Geometry: final body of the model. Coordinates: model frame, mm. A direction names the side the tool comes from. Give positions to 0.01 mm unless a question says otherwise; leave off trailing zeros. Loops run counter-clockwise (first coordinate to the right, second up) from the corner with the lowest first, then second, coordinate; pieces in that order, holes last.
from build123d import *

# Parameters (mm, degrees)
SKETCH1_W           = 419.1
SKETCH1_H           = 142.18412
BOSS_EXTRUDE1_DEPTH = 88.9
SKETCH2_R           = 119.38
CUT_EXTRUDE1_DEPTH  = 83.4009
SKETCH7_W           = 187.160719179
SKETCH7_H           = 30.93974
SKETCH7_H_2         = 43.28668
CUT_EXTRUDE2_DEPTH  = 452.402640644
SKETCH4_R           = 40.386
CUT_EXTRUDE4_DEPTH  = 7.62
CUT_EXTRUDE17_START = -12.7
CUT_EXTRUDE17_DEPTH = 12.7
CUT_EXTRUDE18_DEPTH = 12.7
SKETCH18_R          = 25.527
CUT_EXTRUDE11_DEPTH = 23.09114
SKETCH8_W           = 419.1
SKETCH8_H           = 88.9
CUT_EXTRUDE6_DEPTH  = 7.85114
SKETCH9_W           = 419.1
SKETCH9_H           = 88.9
CUT_EXTRUDE7_DEPTH  = 7.14248
SKETCH10_W          = 219.202
SKETCH10_H          = 88.9
CUT_EXTRUDE8_DEPTH  = 30.48
SKETCH12_W          = 121.533574186
SKETCH12_H          = 96.7105
BOSS_EXTRUDE2_DEPTH = 50.8
SKETCH14_W          = 55.647095764
SKETCH14_H          = 96.7105
BOSS_EXTRUDE3_DEPTH = 12.7
CUT_EXTRUDE10_REACH = 448.907
SKETCH17_R          = 12.827
SKETCH22_W          = 199.898
SKETCH22_H          = 88.9
BOSS_EXTRUDE5_DEPTH = 2.54
SKETCH29_R          = 12.827
CUT_EXTRUDE14_DEPTH = 447.906526346
BOSS_EXTRUDE6_DEPTH = 86.10092
SKETCH45_W          = 107.95
SKETCH45_H          = 50.53076
SKETCH45_H_2        = 15.24
CUT_EXTRUDE22_DEPTH = 452.677672269
SKETCH46_W          = 91.948
SKETCH46_H          = 129.7305
BOSS_EXTRUDE7_DEPTH = 12.7
CUT_EXTRUDE23_DEPTH = 452.677672176


with BuildPart() as part:
    # Sketch1 → Boss-Extrude1 (new body)
    with BuildSketch(Plane(origin=(0, 0, 0), x_dir=(1, 0, 0), z_dir=(0, 1, 0))):
        with Locations((209.55, 71.09206)):
            Rectangle(SKETCH1_W, SKETCH1_H)
    extrude(amount=BOSS_EXTRUDE1_DEPTH)

    # Sketch2 → Cut-Extrude1 (cut)
    with BuildSketch(Plane(origin=(0, 0, -131.63296), x_dir=(-1, 0, 0), z_dir=(0, 0, -1))):
        with Locations((-116.7166499, 150.061217688)):
            Circle(SKETCH2_R)
    extrude(amount=-CUT_EXTRUDE1_DEPTH, mode=Mode.SUBTRACT)

    # Sketch7 → Cut-Extrude2 (cut, through all)
    with BuildSketch(Plane(origin=(0, 88.9, 0), x_dir=(1, 0, 0), z_dir=(0, 1, 0))):
        with Locations((325.519640411, 103.62311)):
            Rectangle(SKETCH7_W, SKETCH7_H)
        with Locations((325.519640411, 33.4899)):
            Rectangle(SKETCH7_W, SKETCH7_H_2)
    extrude(amount=-CUT_EXTRUDE2_DEPTH, mode=Mode.SUBTRACT)

    # Sketch4 → Cut-Extrude4 (cut)
    with BuildSketch(Plane(origin=(0, 0, -67.83324), x_dir=(-1, 0, 0), z_dir=(0, 0, -1))):
        with Locations((-278.649352085, 104.852009966)):
            Circle(SKETCH4_R)
    extrude(amount=CUT_EXTRUDE4_DEPTH, mode=Mode.SUBTRACT)

    # Sketch39 → Cut-Extrude17 (cut)
    with BuildSketch(Plane.XY.offset(-55.13324).offset(CUT_EXTRUDE17_START)):
        with BuildLine():
            Line((231.939280821, 58.527426444), (231.939280821, 88.9))
            Line((231.939280821, 88.9), (342.472006166, 88.9))
            ThreePointArc((342.472006166, 88.9), (296.080170447, 41.417284719), (231.939280821, 58.527426444))
        make_face()
    extrude(amount=CUT_EXTRUDE17_DEPTH, mode=Mode.SUBTRACT)

    # Sketch40 → Cut-Extrude18 (cut)
    with BuildSketch(Plane(origin=(0, 0, -88.15324), x_dir=(-1, 0, 0), z_dir=(0, 0, -1))):
        with BuildLine():
            Line((-231.939280821, 88.9), (-231.939280821, 58.527426444))
            ThreePointArc((-231.939280821, 58.527426444), (-296.080170447, 41.417284719), (-342.472006166, 88.9))
            Line((-342.472006166, 88.9), (-231.939280821, 88.9))
        make_face()
    extrude(amount=-CUT_EXTRUDE18_DEPTH, mode=Mode.SUBTRACT)

    # Sketch18 → Cut-Extrude11 (cut)
    with BuildSketch(Plane(origin=(0, 0, -142.18412), x_dir=(-1, 0, 0), z_dir=(0, 0, -1))):
        with Locations((-278.649352085, 104.852009966)):
            Circle(SKETCH18_R)
    extrude(amount=-CUT_EXTRUDE11_DEPTH, mode=Mode.SUBTRACT)

    # Sketch8 → Cut-Extrude6 (cut)
    with BuildSketch(Plane(origin=(0, 0, -142.18412), x_dir=(-1, 0, 0), z_dir=(0, 0, -1))):
        with Locations((-209.55, 44.45)):
            Rectangle(SKETCH8_W, SKETCH8_H)
    extrude(amount=-CUT_EXTRUDE6_DEPTH, mode=Mode.SUBTRACT)

    # Sketch9 → Cut-Extrude7 (cut)
    with BuildSketch(Plane.XY):
        with Locations((209.55, 44.45)):
            Rectangle(SKETCH9_W, SKETCH9_H)
    extrude(amount=-CUT_EXTRUDE7_DEPTH, mode=Mode.SUBTRACT)

    # Sketch10 → Cut-Extrude8 (cut)
    with BuildSketch(Plane.XY.offset(-7.14248)):
        with Locations((109.601, 44.45)):
            Rectangle(SKETCH10_W, SKETCH10_H)
    extrude(amount=-CUT_EXTRUDE8_DEPTH, mode=Mode.SUBTRACT)

    # Sketch12 → Boss-Extrude2 (add)
    with BuildSketch(Plane.XZ):
        with Locations((-60.766787093, -85.97773)):
            Rectangle(SKETCH12_W, SKETCH12_H)
    extrude(amount=-BOSS_EXTRUDE2_DEPTH)

    # Sketch14 → Boss-Extrude3 (add)
    with BuildSketch(Plane.XZ):
        with Locations((-93.710026304, -85.97773)):
            Rectangle(SKETCH14_W, SKETCH14_H)
    extrude(amount=BOSS_EXTRUDE3_DEPTH)

    # Cut-Extrude10: up to this face of the body (flat: up to its plane)
    cut_extrude10_end = Plane(part.part.faces().sort_by_distance((319.151, 44.45, -7.14248))[0])
    # Sketch17 → Cut-Extrude10 (cut, up to the picked face)
    with BuildSketch(Plane(origin=(0, 0, -134.33298), x_dir=(-1, 0, 0), z_dir=(0, 0, -1)), mode=Mode.PRIVATE) as cut_extrude10_sk1:
        with Locations((-384.735935495, 0.531880938)):
            Circle(SKETCH17_R)
    cut_extrude10_tool1 = split(extrude(cut_extrude10_sk1.sketch, amount=-CUT_EXTRUDE10_REACH, mode=Mode.PRIVATE), bisect_by=cut_extrude10_end, keep=Keep.BOTH, mode=Mode.PRIVATE)
    # Sketch17 → Cut-Extrude10 (cut, up to the picked face)
    with BuildSketch(Plane(origin=(0, 0, -134.33298), x_dir=(-1, 0, 0), z_dir=(0, 0, -1)), mode=Mode.PRIVATE) as cut_extrude10_sk2:
        with Locations((94.798916194, -17.274045482)):
            Circle(SKETCH17_R)
    cut_extrude10_tool2 = split(extrude(cut_extrude10_sk2.sketch, amount=-CUT_EXTRUDE10_REACH, mode=Mode.PRIVATE), bisect_by=cut_extrude10_end, keep=Keep.BOTH, mode=Mode.PRIVATE)
    # Sketch17 → Cut-Extrude10 (cut, up to the picked face)
    with BuildSketch(Plane(origin=(0, 0, -134.33298), x_dir=(-1, 0, 0), z_dir=(0, 0, -1)), mode=Mode.PRIVATE) as cut_extrude10_sk3:
        with BuildLine():
            Line((-169.736021607, 19.31637742), (-169.736021607, 0))
            Line((-169.736021607, 0), (-144.082021607, 0))
            Line((-144.082021607, 0), (-144.082021607, 19.31637742))
            ThreePointArc((-144.082021607, 19.31637742), (-156.909021607, 32.14337742), (-169.736021607, 19.31637742))
        make_face()
    cut_extrude10_tool3 = split(extrude(cut_extrude10_sk3.sketch, amount=-CUT_EXTRUDE10_REACH, mode=Mode.PRIVATE), bisect_by=cut_extrude10_end, keep=Keep.BOTH, mode=Mode.PRIVATE)
    add(cut_extrude10_tool1.solids().sort_by(Axis((384.735935, 0.531881, -134.33298), (0, 0, 1)))[0], mode=Mode.SUBTRACT)
    add(cut_extrude10_tool2.solids().sort_by(Axis((-94.798916, -17.274045, -134.33298), (0, 0, 1)))[0], mode=Mode.SUBTRACT)
    add(cut_extrude10_tool3.solids().sort_by(Axis((156.909022, 14.834778, -134.33298), (0, 0, 1)))[0], mode=Mode.SUBTRACT)

    # Sketch22 → Boss-Extrude5 (add)
    with BuildSketch(Plane.XY.offset(-7.14248)):
        with Locations((319.151, 44.45)):
            Rectangle(SKETCH22_W, SKETCH22_H)
    extrude(amount=BOSS_EXTRUDE5_DEPTH)

    # Sketch29 → Cut-Extrude14 (cut, through all)
    with BuildSketch(Plane(origin=(0, 0, -7.14248), x_dir=(-1, 0, 0), z_dir=(0, 0, -1))):
        with Locations((-384.735935495, 0.531880938)):
            Circle(SKETCH29_R)
    extrude(amount=-CUT_EXTRUDE14_DEPTH, mode=Mode.SUBTRACT)

    # Sketch30 → Boss-Extrude6 (add)
    with BuildSketch(Plane(origin=(0, 0, -134.33298), x_dir=(-1, 0, 0), z_dir=(0, 0, -1))):
        with BuildLine():
            Line((-14.194018979, 88.9), (-20.758717893, 88.9))
            ThreePointArc((-20.758717893, 88.9), (-116.7166499, 36.269217688), (-212.674581906, 88.9))
            Line((-212.674581906, 88.9), (-219.239280821, 88.9))
            ThreePointArc((-219.239280821, 88.9), (-116.7166499, 30.681217688), (-14.194018979, 88.9))
        make_face()
    extrude(amount=-BOSS_EXTRUDE6_DEPTH)

    # Sketch44 → Cut-Revolve1 (revolve, cut)
    with BuildSketch(Plane(origin=(0, 104.852009966, 0), x_dir=(1, 0, 0), z_dir=(0, 1, 0))):
        with BuildLine():
            Line((278.649352085, 11.84656), (306.589352085, 11.84656))
            ThreePointArc((306.589352085, 11.84656), (307.31205993, 7.964449393), (309.383352085, 4.60248))
            Line((309.383352085, 4.60248), (278.649352085, 4.60248))
            Line((278.649352085, 4.60248), (278.649352085, 11.84656))
        make_face()
    revolve(axis=Axis((278.649352085, 104.852009966, -328.456473898), (0, 0, 1)), mode=Mode.SUBTRACT)

    # Sketch45 → Cut-Extrude22 (cut, through all)
    with BuildSketch(Plane(origin=(0, 88.9, 0), x_dir=(1, 0, 0), z_dir=(0, 1, 0))):
        with Locations((365.125, 29.86786)):
            Rectangle(SKETCH45_W, SKETCH45_H)
        with Locations((365.125, 126.71298)):
            Rectangle(SKETCH45_W, SKETCH45_H_2)
    extrude(amount=-CUT_EXTRUDE22_DEPTH, mode=Mode.SUBTRACT)

    # Sketch46 → Boss-Extrude7 (add)
    with BuildSketch(Plane.XZ):
        with Locations((265.176, -69.46773)):
            Rectangle(SKETCH46_W, SKETCH46_H)
    extrude(amount=-BOSS_EXTRUDE7_DEPTH)

    # Sketch47 → Cut-Extrude23 (cut, through all)
    with BuildSketch(Plane(origin=(0, 88.9, 0), x_dir=(1, 0, 0), z_dir=(0, 1, 0))):
        with BuildLine():
            Line((222.900157375, 134.33298), (90.917885838, 134.33298))
            ThreePointArc((90.917885838, 134.33298), (156.909021607, 96.23298), (222.900157375, 134.33298))
        make_face()
    extrude(amount=-CUT_EXTRUDE23_DEPTH, mode=Mode.SUBTRACT)


solid = part.part
Item 1: Draft query along X for faces 5 (the face through (311.15, 35, -121)), 6 (the face through (271, 12.7, -103)), 7 (the face through (-95.02, -4.45, -86.65)). Return one class per face: +X half, -X half, draft (parallel to the pull), parting line (faces both ways), or undercut.
Values follow:
face 5: +X half
face 6: draft
face 7: undercut
Item 2: Section query C-C on z = -27. Return loops of the section in (x, y).
Values follow:
outline: (219.2, 0) - (311.15, 0) - (311.15, 12.7) - (231.94, 12.7) - (231.94, 88.9) - (219.2, 88.9) - close
Item 3: Section query D-D on x = -43. Return loops of the section in (y, z).
Values follow:
outline: (0, -134.33) - (50.8, -134.33) - (50.8, -37.62) - (0, -37.62) - close
Item 4: Section query A-A on z = -102.5. Return loops of the section in (x, y), plus the area to 3 significant figures.
Values follow:
outline: (-121.53, -12.7) - (-106.78, -12.7) arc R12.83 cw to (-82.82, -12.7) - (-65.89, -12.7) - (-65.89, 0) - (126.65, 0) - (126.65, 36.7) arc R113.79 cw to (20.76, 88.9) - (0, 88.9) - (0, 50.8) - (-121.53, 50.8) - close; (187.17, 0) - (311.15, 0) - (311.15, 12.7) - (231.94, 12.7) - (231.94, 88.9) - (212.67, 88.9) arc R113.79 cw to (187.17, 60.7) - close
area: 18,500 mm2
Item 5: Ray query, probe 1 along Z at (x, y) = (232.5, 56); probe 2 along Z at (x, y) = (245, 67); probe 3 along X at (y, z) = (14, -48). Return the intervals inside material, ascending.
Values follow:
probe 1: z = -134.33 to -119.09, -88.15 to -55.13, -11.85 to -4.6
probe 2: z = -134.33 to -119.09, -75.45 to -67.83, -11.85 to -4.6
probe 3: x = -121.53 to 144.08, 169.74 to 231.94
Item 6: Pin query (flat end, axial travel): pin 1 (19 mm diameter, centred on y = 74.5, z = -64.5, fed in from -X); pin 2 (4 mm diameter, centred on y = 28.5, z = -26.5, fed in from +X); pin 3 (4 mm diameter, centred on x = 184.5, z = -46, fed in from -Y). Return the tip coordinate at first contact, or that it passes through.
Values follow:
pin 1: stops at x = 0
pin 2: stops at x = 231.94
pin 3: stops at y = 0
Item 7: Section query B-B on y = 6. Return loops of the section in (x, z).
Values follow:
outline: (-121.53, -134.33) - (90.92, -134.33) arc R76.2 cw to (144.08, -97.32) - (144.08, -37.62) - (-121.53, -37.62) - close; (169.74, -97.32) arc R76.2 cw to (222.9, -134.33) - (311.15, -134.33) - (311.15, -88.15) - (373.13, -88.15) - (373.13, -55.13) - (311.15, -55.13) - (311.15, -4.6) - (219.2, -4.6) - (219.2, -37.62) - (169.74, -37.62) - close; (396.34, -88.15) - (419.1, -88.15) - (419.1, -55.13) - (396.34, -55.13) - close
Item 8: Set-up query: faces 1 (the face through (-62, 50.8, -85)), 2 (the face through (144.082, 10, -68)), 3 (the face through (38, 0, -85)), 4 (the face through (288, 64, -67.833)). Return all of +Z, -Z, +X, -X, +Y, -Y with unobstructed straight access to the full face (end or side cutting, diameter ignored); none if empty.
Values follow:
face 1: +Z, -Z, -X, +Y
face 2: +Z, -Z, -Y
face 3: +Z, -Z, +X, -Y
face 4: +Y
